Check sheet for the drawn part. Datum: minimum x, y, z corner. Units: mm. Coordinates: 2 decimals unless noted, no trailing zeros. Order: outer loops, then holes, each group sorted by start corner. A loop starts at its lowest first (then second) coordinate and runs counter-clockwise, first axis right, second up. Notation, with made-up numbers: (-39.75, 54.5) - (0.25, 54.5) arc R28 ccw to (0.25, 73.5) - close; hole circle Ø6 at (-36.75, 7). An arc over 180 degrees is marked (long way). Return JSON: item names as keys, results as strings. Group by question number.
Item 1: Section check C-C on x = 39. Enter the section's corners in (y, z) (3 decimals).
Item 2: Gauge pin test, flat end, axial feed: pin 1 (1.6 mm diameter, centred on x = 35, y = 2, fed in from -Z) (3 decimals). Record the tip position at first contact, or that the pin passes through.
Item 3: Section check A-A on x = 32. Enter the section's corners in (y, z) (3 decimals), then the cut area to 3 significant figures.
Item 4: Scan lines: probe 1 along Z at (x, y) = (9, 0.25); probe 2 along X at (y, z) = (0.7, 8); probe 3 along Z at (x, y) = (41, 1.2). Record each from-to range of solid material in increasing order.
Item 5: Section check D-D on y = 1.6. Give the number of separate pieces and of enclosed holes in the cut face, then the cut area to 3 significant figures.
Item 6: Section check B-B on z = 15.5. Enter the section's corners in (x, y) (3 decimals).
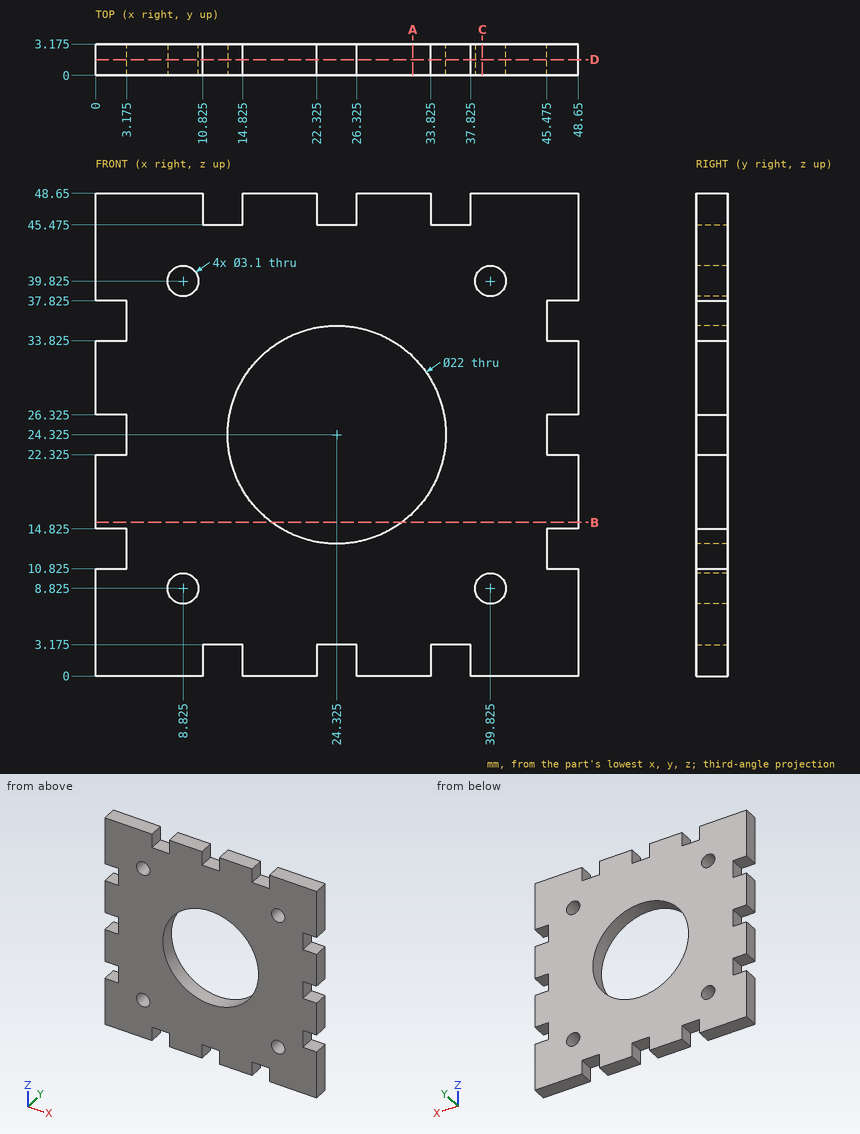
Computed:
{
 "1": {"outline": "(0, 0) - (3.175, 0) - (3.175, 7.513) - (0, 7.513) - close; (0, 10.137) - (3.175, 10.137) - (3.175, 38.513) - (0, 38.513) - close; (0, 41.137) - (3.175, 41.137) - (3.175, 48.65) - (0, 48.65) - close"},
 "2": {"pin 1": "stops at z = 3.175"},
 "3": {"outline": "(0, 0) - (3.175, 0) - (3.175, 16.445) - (0, 16.445) - close; (0, 32.205) - (3.175, 32.205) - (3.175, 48.65) - (0, 48.65) - close", "area": "104 mm²"},
 "4": {"probe 1": "z = 0 to 7.28, 10.37 to 38.28, 41.37 to 48.65", "probe 2": "x = 0 to 7.51, 10.14 to 38.51, 41.14 to 48.65", "probe 3": "z = 0 to 7.81, 9.84 to 38.81, 40.84 to 48.65"},
 "5": {"separate pieces": "1", "enclosed holes": "5", "area": "1,800 mm²"},
 "6": {"outline": "(0, 0) - (17.758, 0) - (17.758, 3.175) - (0, 3.175) - close; (30.892, 0) - (48.65, 0) - (48.65, 3.175) - (30.892, 3.175) - close"}
}
